```python
from build123d import *

# Parameters (mm, degrees)
SKETCH1_R           = 1.75
BOSS_EXTRUDE1_DEPTH = 3
FILLET1_R           = 10


with BuildPart() as part:
    # Sketch1 → Boss-Extrude1 (new body)
    with BuildSketch(Plane.XY):
        with BuildLine():
            Line((0, 43.5), (0, 9.968037932))
            Line((0, 9.968037932), (3.389895868, 5))
            Line((3.389895868, 5), (3.389895868, 2))
            Line((3.389895868, 2), (-4.710104132, 2))
            Line((-4.710104132, 2), (-4.710104132, 5))
            Line((-4.710104132, 5), (-14.510104132, 5))
            Line((-14.510104132, 5), (-14.510104132, 2))
            Line((-14.510104132, 2), (-22.610104132, 2))
            Line((-22.610104132, 2), (-22.610104132, 5))
            Line((-22.610104132, 5), (-19.210104132, 9.968037932))
            Line((-19.210104132, 9.968037932), (-19.210104132, 17.5))
            Line((-19.210104132, 17.5), (-31.5, 17.5))
            ThreePointArc((-31.5, 17.5), (-34.5, 20.5), (-31.5, 23.5))
            Line((-31.5, 23.5), (-24.207476636, 23.5))
            Line((-24.207476636, 23.5), (-24.207476636, 37.5))
            Line((-24.207476636, 37.5), (-31.5, 37.5))
            ThreePointArc((-31.5, 37.5), (-34.5, 40.5), (-31.5, 43.5))
            Line((-31.5, 43.5), (0, 43.5))
        make_face()
        with Locations((-31.5, 40.5)):
            Circle(SKETCH1_R, mode=Mode.SUBTRACT)
        with Locations((-31.5, 20.5)):
            Circle(SKETCH1_R, mode=Mode.SUBTRACT)
    extrude(amount=BOSS_EXTRUDE1_DEPTH)

    # Fillet1
    fillet1_edges = [part.edges().sort_by_distance(p)[0] for p in [
        (0, 43.5, 1.5),
    ]]
    fillet(fillet1_edges, radius=FILLET1_R)


solid = part.part
```
Read the model definition and answer for the solid it produces. Units are mm, in the model's axes. A direction names the side the tool comes from. Round coordinates to 2 decimals unless told otherwise and drop trailing zeros. Write each loop counter-clockwise with the first axis right and the second up, starting at its lowest first coordinate (ties: lowest second). Pieces come first, ordered by that corner, then holes. Notation, with made-up numbers: M -17.5,-31 L 18.5,-31 A30 ccw 18.5,6 Z; hole C 21.25,29 d1. An arc over 180 degrees is marked long. One line per item, written item: value.
Q1. Straight lines are drawn through the part: line 1 (Y direction, x = -31.5, z = 0.9); line 2 (X direction, y = 4, z = 2.4); line 3 (Y direction, x = -28.5, z = 0.4). For each, find the intervals that lie inside material, in ascending order. Write a range as [from, to].
Data:
line 1: [17.5, 18.75], [22.25, 23.5], [37.5, 38.75], [42.25, 43.5]
line 2: [-22.61, -14.51], [-4.71, 3.39]
line 3: [17.5, 23.5], [37.5, 43.5]
Q2. Find section B-B on z = 1.25. Write down the section's boundary in (x, y).
Data:
outline: M -31.5,17.5 L -19.21,17.5 L -19.21,9.97 L -22.61,5 L -22.61,2 L -14.51,2 L -14.51,5 L -4.71,5 L -4.71,2 L 3.39,2 L 3.39,5 L 0,9.97 L 0,33.5 A10 ccw -10,43.5 L -31.5,43.5 A3 ccw -31.5,37.5 L -24.21,37.5 L -24.21,23.5 L -31.5,23.5 A3 ccw Z; hole C -31.5,20.5 d3.5; hole C -31.5,40.5 d3.5
Q3. Flat-ended cylindrical pins translate along their axes: pin 1 Ø3 at (x, y) = (-31.5, 20.5) entering from -Z; pin 2 Ø1.5 at (x, z) = (-28, 2) entering from -Y; pin 3 Ø0.9 at (y, z) = (3.5, 1.5) entering from -X; pin 4 Ø1.5 at (y, z) = (16.5, 1.5) entering from +X. Find the tip coordinate at first contact, or state that the pin passes through.
Data:
pin 1: through
pin 2: y = 17.5
pin 3: x = -22.61
pin 4: x = 0
Q4. Find section A-A on y = 20.5. Write down the section's boundary in (x, z).
Data:
outline: M -34.5,0 L -33.25,0 L -33.25,3 L -34.5,3 Z; M -29.75,0 L 0,0 L 0,3 L -29.75,3 Z
Q5. Find section D-D on y = 29. Write down the section's boundary in (x, z).
Data:
outline: M -24.21,0 L 0,0 L 0,3 L -24.21,3 Z
Q6. Which of the six approach directions +Z, -Z, +X, -X, +Y, -Y give full straight-line access (tool end or side, diameter ignored) to faces 5 (the flat face through (-10, 5, 1)), 6 (the flat face through (-20.934, 7.449, 1.479)), 7 (the flat face through (0, 22, 1))?
Data:
face 5: +Z, -Z, -Y
face 6: +Z, -Z, -X
face 7: +Z, -Z, +X, +Y
Q7. Find section C-C on x = -20.5. Write down the section's boundary in (y, z), plus the area to 4 significant figures.
Data:
outline: M 2,0 L 8.08,0 L 8.08,3 L 2,3 Z; M 17.5,0 L 43.5,0 L 43.5,3 L 17.5,3 Z
area: 96.25 mm2
Q8. For a pull along Y with two mould halves and no side action, classify faces 1 (the flat face through (-1, 2, 1)), 2 (the flat face through (-28, 37.5, 1)), 3 (the flat face through (1.67, 7.52, 1.48)), 4 (the flat face through (3.39, 4, 1)) as +Y half, -Y half, draft (parallel to the pull), parting line (faces both ways), or undercut.
Data:
face 1: -Y half
face 2: undercut
face 3: +Y half
face 4: draft
